Could you check a few things on this drawing? It's one solid part, dimensions in mm from its lowest x, y, z. A direction names the side the tool comes from. Round coordinates to 2 decimals unless told otherwise and drop trailing zeros. Write each loop counter-clockwise with the first axis right and the second up, starting at its lowest first coordinate (ties: lowest second). Pieces come first, ordered by that corner, then holes. Notation, with made-up numbers: (-19, 30) -> (-11, 30) arc R15 cw to (-11, 46) -> close; hole circle Ø8 at (52.25, -8). An arc over 180 degrees is marked (long way). Answer in a Markdown table with one row per item.
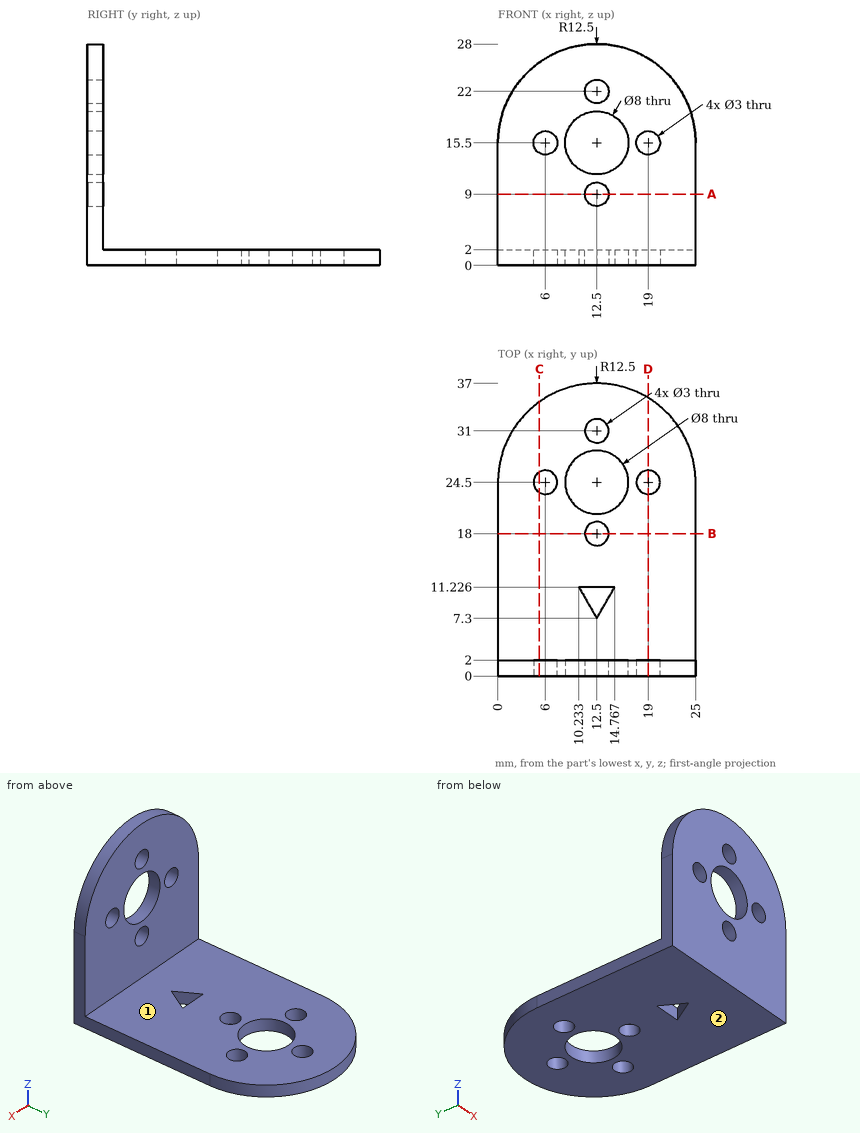
1) Imagine slicing it at C-C, the plane x = 5.25. Please give me the cut outline in (y, z).
Findings:
| item | result |
|---|---|
| outline | (0, 0) -> (23.2, 0) -> (23.2, 2) -> (2, 2) -> (2, 14.2) -> (0, 14.2) -> close; (0, 16.8) -> (2, 16.8) -> (2, 25.68) -> (0, 25.68) -> close; (25.8, 0) -> (34.68, 0) -> (34.68, 2) -> (25.8, 2) -> close |
2) For pin 1 (7 mm diameter, centred on x = 12.5, z = 15.5, fed in from -Y); pin 2 (3 mm diameter, centred on x = 16, y = 17, fed in from +Z); pin 3 (5 mm diameter, centred on x = 17, y = 4, fed in from +Z) (1 decimal); pin 4 (2 mm diameter, centred on x = 7.5, z = 6, fed in from +Y), each with a flat end and sliding along its axis, tell me the tip position at first contact or that it passes through.
Findings:
| item | result |
|---|---|
| pin 1 | passes through |
| pin 2 | stops at z = 2 |
| pin 3 | stops at z = 27.6 |
| pin 4 | stops at y = 2 |
3) For the marked faces 1 and 2, which set-ups out of +Z, -Z, +X, -X, +Y, -Y let a thin tool reach every point of the face, with its end or its side?
Findings:
| item | result |
|---|---|
| face 1 | +Z, +X, -X, +Y |
| face 2 | -Z, +X, -X, +Y, -Y |
4) Imagine slicing it at A-A, the plane z = 9. Please give me the cut outline in (x, y), plus the area to 3 significant figures.
Findings:
| item | result |
|---|---|
| outline | (0, 0) -> (11, 0) -> (11, 2) -> (0, 2) -> close; (14, 0) -> (25, 0) -> (25, 2) -> (14, 2) -> close |
| area | 44.0 mm^2 |
5) Please list where these lines run through material, in increasing order: line 1 (Z direction, x = 12.5, y = 1.15); line 2 (Y direction, x = 15.75, z = 5).
Findings:
| item | result |
|---|---|
| line 1 | z = 0 to 7.5, 10.5 to 11.5, 19.5 to 20.5, 23.5 to 28 |
| line 2 | y = 0 to 2 |
6) Imagine slicing it at D-D, the plane x = 19. Please give me the cut outline in (y, z).
Findings:
| item | result |
|---|---|
| outline | (0, 0) -> (23, 0) -> (23, 2) -> (2, 2) -> (2, 14) -> (0, 14) -> close; (0, 17) -> (2, 17) -> (2, 26.18) -> (0, 26.18) -> close; (26, 0) -> (35.18, 0) -> (35.18, 2) -> (26, 2) -> close |
